Could you check a few things on this drawing? It's one solid part, dimensions in mm from its lowest x, y, z. A direction names the side the tool comes from. Coordinates: 2 decimals unless noted, no trailing zeros. Loops run counter-clockwise (first coordinate to the right, second up) from the corner with the lowest first, then second, coordinate; pieces in that order, holes last. Notation, with made-up numbers: M 79,85.5 L 118,85.5 A21 ccw 118,120.5 Z; hole C 1.5,48.5 d2. An arc over 180 degrees is marked long. Use one line per item in the form item = value. Start each with the question number.
(1) Will these pins go through, and if not, where does the flat tip stop? P1, Ø7, axis at x = 7.5, z = 13, coming from the -Y side; P2, Ø1, axis at x = 5.5, z = 3.5, coming from the -Y side; P3, Ø3, axis at x = 4.5, z = 6.5, coming from the +Y side; P4, Ø3, axis at x = 7.5, z = 7, coming from the -Y side.
(2) Please list where these lines run through material, in increasing order: L1, parallel to Z at x = 7.5, y = 9.75; L2, parallel to Z at x = 12.75, y = 6.25; L3, parallel to X at y = 8, z = 13.
(3) Imagine slicing it at A-A, the plane x = 7.5. Please give me the cut outline in (y, z), and give its area (3 significant figures).
(4) Imagine slicing it at C-C, the plane y = 7.5. Please give me the cut outline in (x, z).
(5) Imagine slicing it at D-D, the plane z = 10.75. Please give me the cut outline in (x, y), and give its area (3 significant figures).
(6) Imagine slicing it at B-B, the plane y = 3.75. Please give me the cut outline in (x, z), and give its area (3 significant figures).
(7) Thinking about a two-plate mould opening in X: for the marked faces 3, 4 and 5, which applies, +X half, -X half, draft (parallel to the pull), parting line (faces both ways), or undercut?
(8) On a 3-axis mill with a long thin cutter (end or side, diameter ignored), from which of +Z, -Z, +X, -X, +Y, -Y can I reach the whole of each face in a straight line? I mean the marked faces 1 and 2. Say none if no direction works.
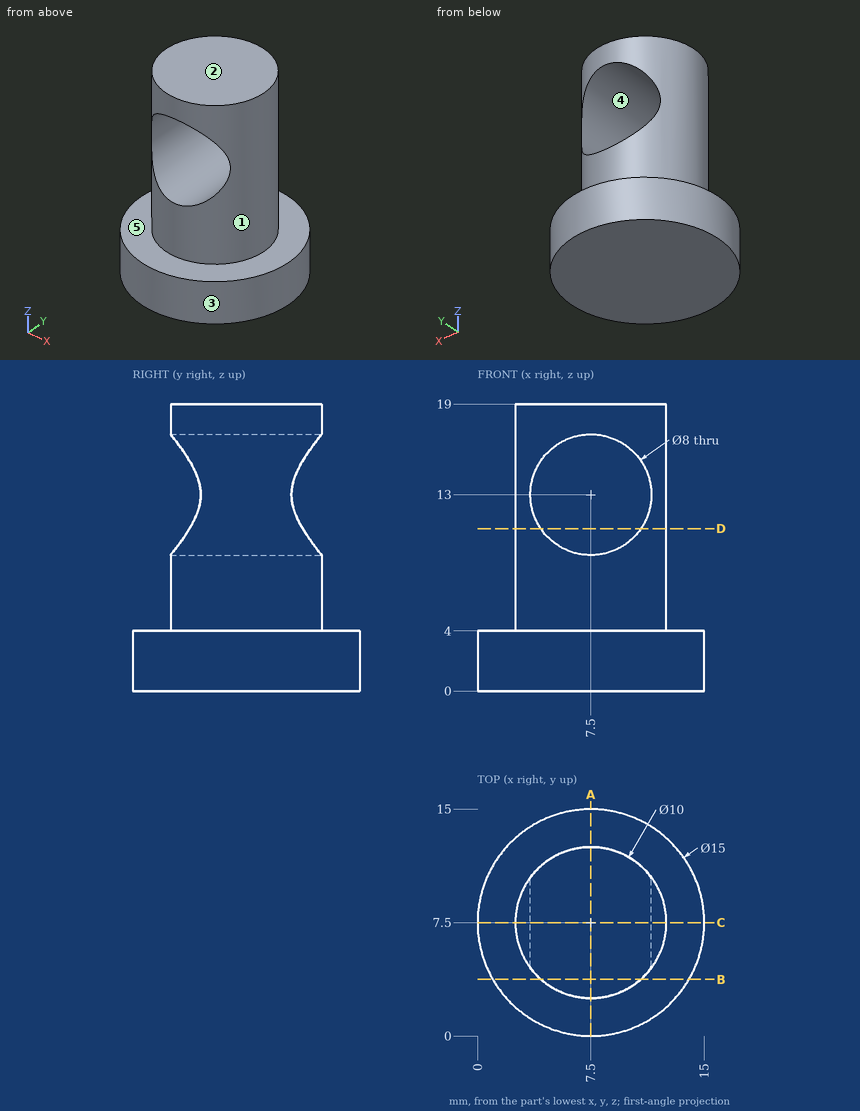
Answer:
q1.P1 = through
q1.P2 = 0.15
q1.P3 = 12.27
q1.P4 = 2.5
q2.L1 = 0 to 9, 17 to 19
q2.L2 = 0 to 4
q2.L3 = 2.53 to 3.5, 11.5 to 12.47
q3.outline = M 0,0 L 15,0 L 15,4 L 12.5,4 L 12.5,9 L 2.5,9 L 2.5,4 L 0,4 Z; M 2.5,17 L 12.5,17 L 12.5,19 L 2.5,19 Z
q3.area = 130 mm²
q4.outline = M 0,0 L 15,0 L 15,4 L 12.5,4 L 12.5,19 L 2.5,19 L 2.5,4 L 0,4 Z; hole C 7.5,13 d8
q5.outline = M 4.19,3.75 L 4.19,11.25 A5 ccw Z; M 10.81,3.75 A5 ccw 10.81,11.25 Z
q5.area = 17.6 mm²
q6.outline = M 1,0 L 14,0 L 14,4 L 10.81,4 L 10.81,10.75 A4 cw 4.19,10.75 L 4.19,4 L 1,4 Z; M 4.19,15.25 A4 cw 10.81,15.25 L 10.81,19 L 4.19,19 Z
q6.area = 105 mm²
q7.face_3 = parting line
q7.face_4 = undercut
q7.face_5 = draft
q8.face_1 = +Z
q8.face_2 = +Z, +X, -X, +Y, -Y
